Part model, mm, in its own coordinate system. Coordinates: 2 decimals unless noted, no trailing zeros. Loops run counter-clockwise (first coordinate to the right, second up) from the corner with the lowest first, then second, coordinate; pieces in that order, holes last. Notation, with made-up numbers: (-38, 31.5) - (11, 31.5) arc R27 cw to (11, 68.5) - close; hole circle Ø9 at (-1.75, 77.25). An arc over 180 degrees is marked (long way). Answer as CSV lines item,"result".
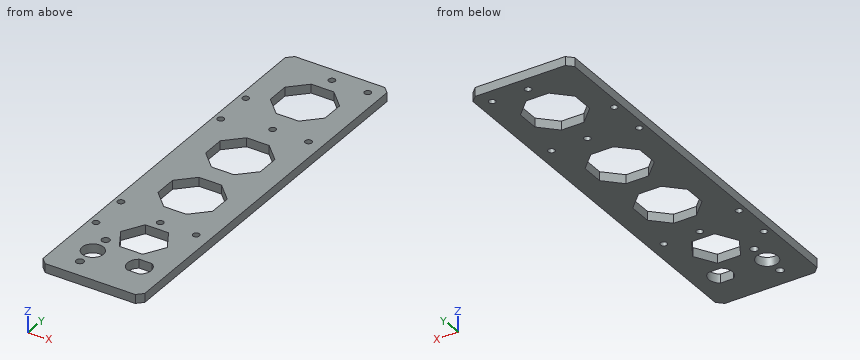
from build123d import *

# Parameters (mm, degrees)
CROQUIS1_W                   = 200
CROQUIS1_H                   = 52.5
SALIENTE_EXTRUIR1_DEPTH      = 4.6
CORTAR_EXTRUIR1_REACH        = 105.49
CORTAR_EXTRUIR2_REACH        = 105.49
CROQUIS3_R                   = 5.5
CROQUIS3_R_2                 = 2
TALADRO_DE_MARGEN_PARA_M31_D = 3.4
CHAFL_N1_SIZE                = 3
TALADRO_DE_MARGEN_PARA_M32_D = 3.4
CORTAR_EXTRUIR3_DEPTH        = 10


with BuildPart() as part:
    # Croquis1 → Saliente-Extruir1 (new body)
    with BuildSketch(Plane(origin=(0, 0, 0), x_dir=(0, 1, 0), z_dir=(0, 0, 1))):
        Rectangle(CROQUIS1_W, CROQUIS1_H)
    extrude(amount=SALIENTE_EXTRUIR1_DEPTH)

    # Croquis2 → Cortar-Extruir1 (cut, up to next)
    with BuildSketch(Plane.XY.offset(4.6), mode=Mode.PRIVATE) as cortar_extruir1_sk1:
        with BuildLine():
            Line((9.16833375, -74.95), (15.83166625, -74.95))
            ThreePointArc((15.83166625, -74.95), (18.55, -80), (15.83166625, -85.05))
            Line((15.83166625, -85.05), (9.16833375, -85.05))
            ThreePointArc((9.16833375, -85.05), (6.45, -80), (9.16833375, -74.95))
        make_face()
    cortar_extruir1_tool1 = extrude(cortar_extruir1_sk1.sketch, amount=-CORTAR_EXTRUIR1_REACH, mode=Mode.PRIVATE) & part.part
    add(cortar_extruir1_tool1.solids().sort_by_distance((12.5, -80, 4.6))[0], mode=Mode.SUBTRACT)

    # Croquis3 → Cortar-Extruir2 (cut, up to next)
    with BuildSketch(Plane.XY.offset(4.6), mode=Mode.PRIVATE) as cortar_extruir2_sk1:
        with Locations((-11.5, -80)):
            Circle(CROQUIS3_R)
    cortar_extruir2_tool1 = extrude(cortar_extruir2_sk1.sketch, amount=-CORTAR_EXTRUIR2_REACH, mode=Mode.PRIVATE) & part.part
    # Croquis3 → Cortar-Extruir2 (cut, up to next)
    with BuildSketch(Plane.XY.offset(4.6), mode=Mode.PRIVATE) as cortar_extruir2_sk2:
        with Locations((-11.5, -90.3)):
            Circle(CROQUIS3_R_2)
    cortar_extruir2_tool2 = extrude(cortar_extruir2_sk2.sketch, amount=-CORTAR_EXTRUIR2_REACH, mode=Mode.PRIVATE) & part.part
    # Croquis3 → Cortar-Extruir2 (cut, up to next)
    with BuildSketch(Plane.XY.offset(4.6), mode=Mode.PRIVATE) as cortar_extruir2_sk3:
        with Locations((-11.5, -69.7)):
            Circle(CROQUIS3_R_2)
    cortar_extruir2_tool3 = extrude(cortar_extruir2_sk3.sketch, amount=-CORTAR_EXTRUIR2_REACH, mode=Mode.PRIVATE) & part.part
    add(cortar_extruir2_tool1.solids().sort_by_distance((-11.5, -80, 4.6))[0], mode=Mode.SUBTRACT)
    add(cortar_extruir2_tool2.solids().sort_by_distance((-11.5, -90.3, 4.6))[0], mode=Mode.SUBTRACT)
    add(cortar_extruir2_tool3.solids().sort_by_distance((-11.5, -69.7, 4.6))[0], mode=Mode.SUBTRACT)

    # Taladro de margen para M31 (through all)
    with Locations(Plane(origin=(0, 0, 0), x_dir=(1, 0, 0), z_dir=(0, 0, -1))):
        with Locations((19.25, -45), (19.25, 45), (0.75, 45), (0.75, -45), (19.25, -92.5), (0.75, -92.5)):
            Hole(TALADRO_DE_MARGEN_PARA_M31_D / 2)

    # Chafl_n1
    chafl_n1_edges = [part.edges().sort_by_distance(p)[0] for p in [
        (26.25, 100, 2.3),
        (26.25, -100, 2.3),
        (-26.25, -100, 2.3),
        (-26.25, 100, 2.3),
    ]]
    chamfer(chafl_n1_edges, length=CHAFL_N1_SIZE)

    # Taladro de margen para M32 (through all)
    with Locations(Plane.XY.offset(4.6)):
        with Locations((-22.75, -60), (-22.75, -40), (-22.75, 40), (-22.75, 60)):
            Hole(TALADRO_DE_MARGEN_PARA_M32_D / 2)

    # Croquis8 → Cortar-Extruir3 (cut)
    with BuildSketch(Plane(origin=(0, 0, 0), x_dir=(1, 0, 0), z_dir=(0, 0, -1))):
        Polygon((-5.090411229, 33.2), (-13.35, 24.940411229), (-13.35, 13.259588771), (-5.090411229, 5), (6.590411229, 5), (14.85, 13.259588771), (14.85, 24.940411229), (6.590411229, 33.2), align=None)
        Polygon((6.590411229, -33.2), (-5.090411229, -33.2), (-13.35, -24.940411229), (-13.35, -13.259588771), (-5.090411229, -5), (6.590411229, -5), (14.85, -13.259588771), (14.85, -24.940411229), align=None)
        Polygon((-5.090411229, -56.8), (-13.35, -65.059588771), (-13.35, -76.740411229), (-5.090411229, -85), (6.590411229, -85), (14.85, -76.740411229), (14.85, -65.059588771), (6.590411229, -56.8), align=None)
        Polygon((-3.749578543, 50), (8.249578543, 50), (14.249157087, 60.391574861), (8.249578543, 70.783149723), (-3.749578543, 70.783149723), (-9.749157087, 60.391574861), align=None)
    extrude(amount=-CORTAR_EXTRUIR3_DEPTH, mode=Mode.SUBTRACT)


solid = part.part
Q1. Saw through at A-A (y = -90.3). Give the cut face in (x, z), then the cut area to 3 significant figures.
Results:
outline,"(-26.25, 0) - (-13.5, 0) - (-13.5, 4.6) - (-26.25, 4.6) - close; (-9.5, 0) - (26.25, 0) - (26.25, 4.6) - (-9.5, 4.6) - close"
area,"223 mm^2"
Q2. Saw through at D-D (x = -11.5). Give the cut face in (y, z), then the cut area to 3 significant figures.
Results:
outline,"(-100, 0) - (-92.3, 0) - (-92.3, 4.6) - (-100, 4.6) - close; (-88.3, 0) - (-85.5, 0) - (-85.5, 4.6) - (-88.3, 4.6) - close; (-74.5, 0) - (-71.7, 0) - (-71.7, 4.6) - (-74.5, 4.6) - close; (-67.7, 0) - (-26.79, 0) - (-26.79, 4.6) - (-67.7, 4.6) - close; (-11.41, 0) - (11.41, 0) - (11.41, 4.6) - (-11.41, 4.6) - close; (26.79, 0) - (63.21, 0) - (63.21, 4.6) - (26.79, 4.6) - close; (78.59, 0) - (100, 0) - (100, 4.6) - (78.59, 4.6) - close"
area,"620 mm^2"
Q3. Flat gauge pins, fed straight in: pin 1 (1 mm diameter, centred on x = -8, y = -8, fed in from -Z); pin 2 (10 mm diameter, centred on x = -11.5, y = -80, fed in from -Z). Where does each tip first touch, or does it go through?
Results:
pin 1,"stops at z = 0"
pin 2,"passes through"
Q4. Saw through at C-C (y = 92.5). Give the cut face in (x, z).
Results:
outline,"(-26.25, 0) - (-0.95, 0) - (-0.95, 4.6) - (-26.25, 4.6) - close; (2.45, 0) - (17.55, 0) - (17.55, 4.6) - (2.45, 4.6) - close; (20.95, 0) - (26.25, 0) - (26.25, 4.6) - (20.95, 4.6) - close"
Q5. Saw through at B-B (x = 0.75). Count the separate pieces of the cut face and the enclosed holes in it, then the cut area to 3 significant figures.
Results:
separate pieces,"8"
enclosed holes,"0"
area,"388 mm^2"
Q6. Wall check: L1, parallel to Y at x = 19.25, z = 2.45; L2, parallel to Y at x = -22.75, z = 1.3; L3, parallel to X at y = -45, z = 1.6. Give the ranges that are in metal, low to high.
Results:
L1,"y = -100 to -46.7, -43.3 to 43.3, 46.7 to 90.8, 94.2 to 100"
L2,"y = -100 to -61.7, -58.3 to -41.7, -38.3 to 38.3, 41.7 to 58.3, 61.7 to 100"
L3,"x = -26.25 to -0.95, 2.45 to 17.55, 20.95 to 26.25"
